Job drawing, mm, ordinate dimensions from the low corner. One solid piece. Give positions to 0.01 mm unless a question says otherwise; leave off trailing zeros. Order: outer loops, then holes, each group sorted by start corner. A loop starts at its lowest first (then second) coordinate and runs counter-clockwise, first axis right, second up. Notation, with made-up numbers: (18, -16.75) - (55, -16.75) arc R17 cw to (55, -0.75) - close; hole circle Ø8 at (-20.75, 57). An arc over 180 degrees is marked (long way). One line per item, written item: value.
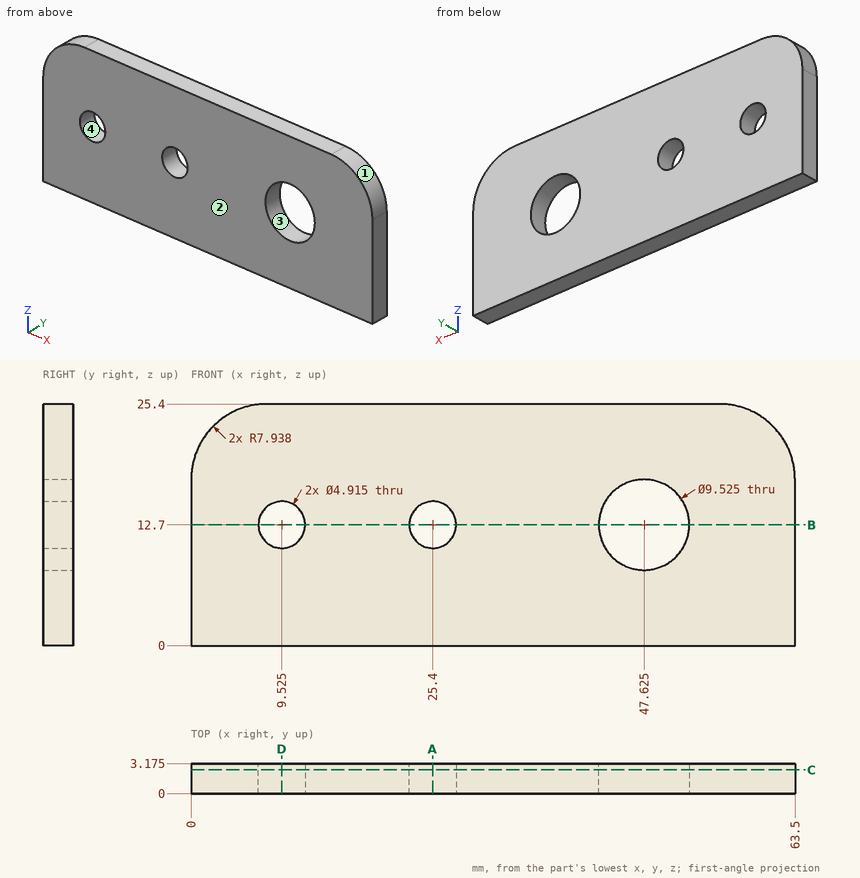
1) Drop flat-ended pins along their axis: P1, Ø1.5, axis at y = 2.5, z = 20.5, coming from the +X side; P2, Ø1.5, axis at y = 1.5, z = 22.5, coming from the -X side. Give the stop position or say it passes through.
Answer:
P1: stops at x = 63.16
P2: stops at x = 1.26
2) Slice it at C-C on y = 2.5. Write the cut outline in (x, z) (1 decimal).
Answer:
outline: (0, 0) - (63.5, 0) - (63.5, 17.5) arc R7.9 ccw to (55.6, 25.4) - (7.9, 25.4) arc R7.9 ccw to (0, 17.5) - close; hole circle Ø4.9 at (9.5, 12.7); hole circle Ø4.9 at (25.4, 12.7); hole circle Ø9.5 at (47.6, 12.7)
3) Wall check: line 1 along X through (y, z) = (2.8, 13) (1 decimal); line 2 along X through (y, z) = (3.05, 14) (1 decimal); line 3 along Z through (x, y) = (44, 1.95). Give the ranges that are in metal, low to high. Write a range as [from, to].
Answer:
line 1: x = [0, 7.1], [12, 23], [27.8, 42.9], [52.4, 63.5]
line 2: x = [0, 7.4], [11.6, 23.3], [27.5, 43], [52.2, 63.5]
line 3: z = [0, 9.61], [15.79, 25.4]
4) Slice it at A-A on x = 25.4. Write the cut outline in (y, z) (1 decimal).
Answer:
outline: (0, 0) - (3.2, 0) - (3.2, 10.2) - (0, 10.2) - close; (0, 15.2) - (3.2, 15.2) - (3.2, 25.4) - (0, 25.4) - close
5) Slice it at B-B on z = 12.7. Write the cut outline in (x, y) (1 decimal).
Answer:
outline: (0, 0) - (7.1, 0) - (7.1, 3.2) - (0, 3.2) - close; (12, 0) - (22.9, 0) - (22.9, 3.2) - (12, 3.2) - close; (27.9, 0) - (42.9, 0) - (42.9, 3.2) - (27.9, 3.2) - close; (52.4, 0) - (63.5, 0) - (63.5, 3.2) - (52.4, 3.2) - close
6) Two-plate mould, pull along X, no slides. Class the marked faces 1, 2, 3 and 4: pulls with the +X half, pulls with the -X half, needs draft (parallel to the pull), parting line crosses it, or undercut.
Answer:
face 1: pulls with the +X half
face 2: needs draft
face 3: undercut
face 4: undercut
